Geometry check sheet. Reference: the model listing, model coordinates, mm. Face numbers are marked on the shaded views. A direction names the side the tool comes from. Give positions to 0.01 mm unless a question says otherwise; leave off trailing zeros. Write each loop counter-clockwise with the first axis right and the second up, starting at its lowest first coordinate (ties: lowest second). Pieces come first, ordered by that corner, then holes. Notation, with made-up numbers: (-38.5, 50.25) - (-28.5, 50.25) arc R23 ccw to (-28.5, 82.25) - close; hole circle Ø7 at (-8.75, -6). An arc over 180 degrees is marked (long way). Use a Markdown table: item, result.
Autodesk Inventor part; units mm, degrees
ref_plane "YZ Plane" through (0, 0, 0) normal (1, 0, 0) x (0, 1, 0)
ref_plane "XZ Plane" through (0, 0, 0) normal (0, 1, 0) x (-1, 0, 0)
ref_plane "XY Plane" through (0, 0, 0) normal (0, 0, 1) x (1, 0, 0)
sketch "スケッチ1" plane through (0, 0, 0) normal (1, 0, 0) x (0, 1, 0)
  line L0 (9, 0) -> (-9, 0) construction
  line L1 (9, 3) -> (-9, 3)
  line L2 (-9, -3) -> (9, -3)
  arc A0 (9, -3) -> (9, 3) centre (9, 0) ccw
  arc A1 (-9, 3) -> (-9, -3) centre (-9, 0) ccw
  line L3 (3, 7) -> (-3, 7)
  line L4 (-3, -7) -> (3, -7)
  line L5 (3, 7) -> (-3, -7) construction
  line L6 (-3, 7) -> (3, -7) construction
  line L7 (-3, 7) -> (-3, 5)
  line L8 (3, 5) -> (3, 7)
  line L9 (3, -7) -> (3, -5)
  line L10 (3, -3) -> (3, 3)
  line L11 (-3, 3) -> (-3, -3)
  line L12 (-3, -5) -> (-3, -7)
  circle A2 centre (-9, 0) radius 1.25
  circle A3 centre (9, 0) radius 1.25
  line L13 (3, -5) -> (3, -3)
  line L14 (3, 3) -> (3, 5)
  line L15 (-3, 5) -> (-3, 3)
  line L16 (-3, -3) -> (-3, -5)
  point P0 (0, 0)
  dimension "d0" = 6
  dimension "d1" = 6
  dimension "d3" = 14
  dimension "d4" = 18
  dimension "d7" = 0
  dimension "d8" = 6
  dimension "d9" = 4
  dimension "d11" = 2.5
  dimension "d12" = 2.5
extrude "押し出し1" add sketch "スケッチ1" along normal blind 3 contours A0 L2 L10 L1 | L10 L2 L11 L1 | L1 L15 L7 L3 L8 L14 | L11 L2 A1 L1 | L13 L9 L4 L12 L16 L2 | A2 | A3
sketch "スケッチ2" plane through (0, 0, 0) normal (-1, 0, 0) x (0, 0, 1)
  spline S0 degree 3 poles (-3.8743, -1.25) (-3.891, -1.25) (-3.9108, -1.2467) (-3.9405, -1.236) (-3.956, -1.2272) (-3.9769, -1.209) (-3.9865, -1.1969) (-3.9969, -1.1748) (-4, -1.1615) (-4, -1.15) knots -0.016775 -0.016775 -0.016775 -0.016775 -0.011755 -0.011755 -0.007303 -0.007303 -0.003437 -0.003437 0 0 0 0
  line L0 (-4, -1.15) -> (-4, 1.15)
  spline S1 degree 3 poles (-4, 1.15) (-4, 1.1615) (-3.9969, 1.1748) (-3.9865, 1.1969) (-3.9769, 1.209) (-3.956, 1.2272) (-3.9405, 1.236) (-3.9108, 1.2467) (-3.891, 1.25) (-3.8743, 1.25) knots 0 0 0 0 0.003437 0.003437 0.007303 0.007303 0.011755 0.011755 0.016775 0.016775 0.016775 0.016775
  line L1 (-3.8743, 1.25) -> (-3.1638, 1.25)
  line L2 (-3.1638, 1.25) -> (-3.1638, 0.47)
  spline S2 degree 3 poles (-3.1638, 0.47) (-3.2063, 0.4464) (-3.2462, 0.4188) (-3.3386, 0.3411) (-3.3965, 0.2704) (-3.4581, 0.1426) (-3.4766, 0.0658) (-3.4766, 0) (-3.4766, -0.0658) (-3.4581, -0.1426) (-3.3965, -0.2704) (-3.3386, -0.3411) (-3.2462, -0.4188) (-3.2063, -0.4464) (-3.1638, -0.47) knots -0.055942 -0.055942 -0.055942 -0.055942 -0.042582 -0.042582 -0.019736 -0.019736 0 0 0 0.019736 0.019736 0.042582 0.042582 0.055942 0.055942 0.055942 0.055942
  line L3 (-3.1638, -0.47) -> (-3.1638, -1.25)
  line L4 (-3.1638, -1.25) -> (-3.8743, -1.25)
  spline S3 degree 3 poles (4, -1.15) (4, -1.1615) (3.9969, -1.1748) (3.9865, -1.1969) (3.9769, -1.209) (3.956, -1.2272) (3.9405, -1.236) (3.9108, -1.2467) (3.891, -1.25) (3.8743, -1.25) knots 0 0 0 0 0.003437 0.003437 0.007303 0.007303 0.011755 0.011755 0.016775 0.016775 0.016775 0.016775
  line L5 (3.8743, -1.25) -> (3.1638, -1.25)
  line L6 (3.1638, -1.25) -> (3.1638, -0.47)
  spline S4 degree 3 poles (3.1638, -0.47) (3.2063, -0.4464) (3.2462, -0.4188) (3.3386, -0.3411) (3.3965, -0.2704) (3.4581, -0.1426) (3.4766, -0.0658) (3.4766, 0) (3.4766, 0.0658) (3.4581, 0.1426) (3.3965, 0.2704) (3.3386, 0.3411) (3.2462, 0.4188) (3.2063, 0.4464) (3.1638, 0.47) knots -0.055942 -0.055942 -0.055942 -0.055942 -0.042582 -0.042582 -0.019736 -0.019736 0 0 0 0.019736 0.019736 0.042582 0.042582 0.055942 0.055942 0.055942 0.055942
  line L7 (3.1638, 0.47) -> (3.1638, 1.25)
  line L8 (3.1638, 1.25) -> (3.8743, 1.25)
  spline S5 degree 3 poles (3.8743, 1.25) (3.891, 1.25) (3.9108, 1.2467) (3.9405, 1.236) (3.956, 1.2272) (3.9769, 1.209) (3.9865, 1.1969) (3.9969, 1.1748) (4, 1.1615) (4, 1.15) knots -0.016775 -0.016775 -0.016775 -0.016775 -0.011755 -0.011755 -0.007303 -0.007303 -0.003437 -0.003437 0 0 0 0
  line L9 (4, 1.15) -> (4, -1.15)
  circle A0 centre (0, 9) radius 1.25
  circle A1 centre (0, -9) radius 1.25
  line L10 (-3, 3) -> (-7, 3)
  line L11 (-7, 3) -> (-7, -3)
  line L12 (-7, -3) -> (-3, -3)
  line L13 (-3, -3) -> (-3, -9)
  arc A2 (-3, -9) -> (3, -9) centre (0, -9) ccw
  line L14 (3, -9) -> (3, -3)
  line L15 (3, -3) -> (7, -3)
  line L16 (7, -3) -> (7, 3)
  line L17 (7, 3) -> (3, 3)
  line L18 (3, 3) -> (3, 9)
  arc A3 (3, 9) -> (-3, 9) centre (0, 9) ccw
  line L19 (-3, 9) -> (-3, 3)
  line L20 (-7, 2.5) -> (-4, 2.2)
  line L21 (-4, 2.2) -> (4, 2.2)
  line L22 (4, 2.2) -> (7, 2.5)
  arc A4 (-3, 3) -> (-3, 5) centre (-3, 4) ccw
  arc A5 (3, 5) -> (3, 3) centre (3, 4) ccw
  line L23 (3, 3) -> (3, 9)
  line L24 (-3, 9) -> (-3, 3)
  point P0 (0, 0)
  point P1 (0, 2.2)
  dimension "d15" = 2
  dimension "d17" = 8
  dimension "d18" = 0.8
  dimension "d19" = 0.5
extrude "押し出し4" cut sketch "スケッチ2" against normal through all contours A4 L19 A3 L18 A5 L17 L16 L22 L21 L20 L11 L10 keep common part
properties part number "tip2" material "アルミニウム 2014-T4"
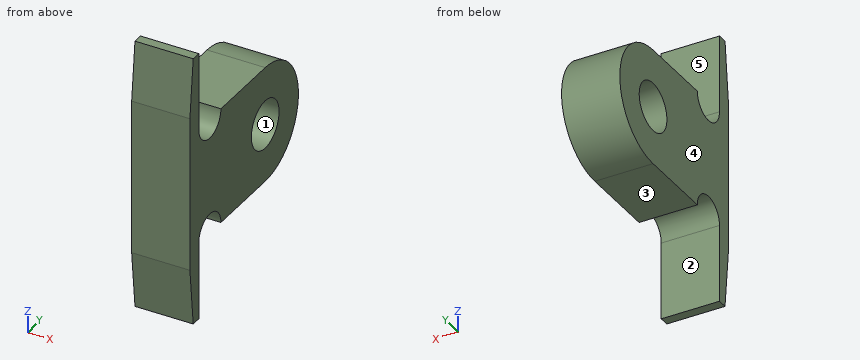
1) Depth check by flat-ended pin: P1, Ø0.9, axis at x = 1.5, y = 7, coming from the +Z side; P2, Ø2, axis at y = 9, z = 0, coming from the +X side; P3, Ø0.9, axis at x = 1.5, y = 6.5, coming from the -Z side; P4, Ø1, axis at x = 1.5, y = 10.5, coming from the +Z side. Enter the tip coordinate at first touch or a pass-through.
Working result:
| item | result |
|---|---|
| P1 | stops at z = 3 |
| P2 | passes through |
| P3 | stops at z = -3 |
| P4 | stops at z = 2.83 |
2) Set-up check for the marked faces 4 and 5: record each of +Z, -Z, +X, -X, +Y, -Y from which the full face is reachable in a straight line by a thin tool's end or side.
Working result:
| item | result |
|---|---|
| face 4 | +Z, -Z, -X, +Y, -Y |
| face 5 | +Z, +X, -X, +Y |
3) Section check B-B on x = 0.35. Record the boundary of the cut face in (y, z), then the cut area to 3 significant figures.
Working result:
| item | result |
|---|---|
| outline | (2.2, -4) - (2.5, -7) - (3, -7) - (3, -3) arc R1 cw to (5, -3) - (9, -3) arc R3 ccw to (9, 3) - (5, 3) arc R1 cw to (3, 3) - (3, 7) - (2.5, 7) - (2.2, 4) - close; hole circle Ø2.5 at (9, 0) |
| area | 52.4 mm² |
4) Mould release check, pull along Y, two halves, no side actions. Record for the marked faces 1, 2 and 3: pulls with the +Y half, pulls with the -Y half, needs draft (parallel to the pull), parting line crosses it, or undercut.
Working result:
| item | result |
|---|---|
| face 1 | undercut |
| face 2 | pulls with the +Y half |
| face 3 | needs draft |
5) Section check C-C on y = 8.5. Record the boundary of the cut face in (x, z), then the cut area to 3 significant figures.
Working result:
| item | result |
|---|---|
| outline | (0, -3) - (3, -3) - (3, -1.15) - (0, -1.15) - close; (0, 1.15) - (3, 1.15) - (3, 3) - (0, 3) - close |
| area | 11.1 mm² |
6) Section check A-A on z = 0. Record the boundary of the cut face in (x, y), then the cut area to 3 significant figures.
Working result:
| item | result |
|---|---|
| outline | (0, 2.2) - (3, 2.2) - (3, 7.75) - (0, 7.75) - close; (0, 10.25) - (3, 10.25) - (3, 12) - (0, 12) - close |
| area | 21.9 mm² |
7) Section check D-D on y = 6.25. Record the boundary of the cut face in (x, z).
Working result:
| item | result |
|---|---|
| outline | (0, -3) - (3, -3) - (3, 3) - (0, 3) - close |
8) Material ranges on L1, parallel to Y at x = 1.1, z = 0; L2, parallel to Z at x = 0.95, y = 6.75; L3, parallel to Y at x = 2.7, z = -3.25, recorded low to high. Write a range as from..to.
Working result:
| item | result |
|---|---|
| L1 | y = 2.2..7.75, 10.25..12 |
| L2 | z = -3..3 |
| L3 | y = 2.2..3 |
